Here's the drawing with two shaded views (mm, measured from the low corner). I have some questions. Coordinates: 2 decimals unless noted, no trailing zeros. Loops run counter-clockwise (first coordinate to the right, second up) from the corner with the lowest first, then second, coordinate; pieces in that order, holes last.
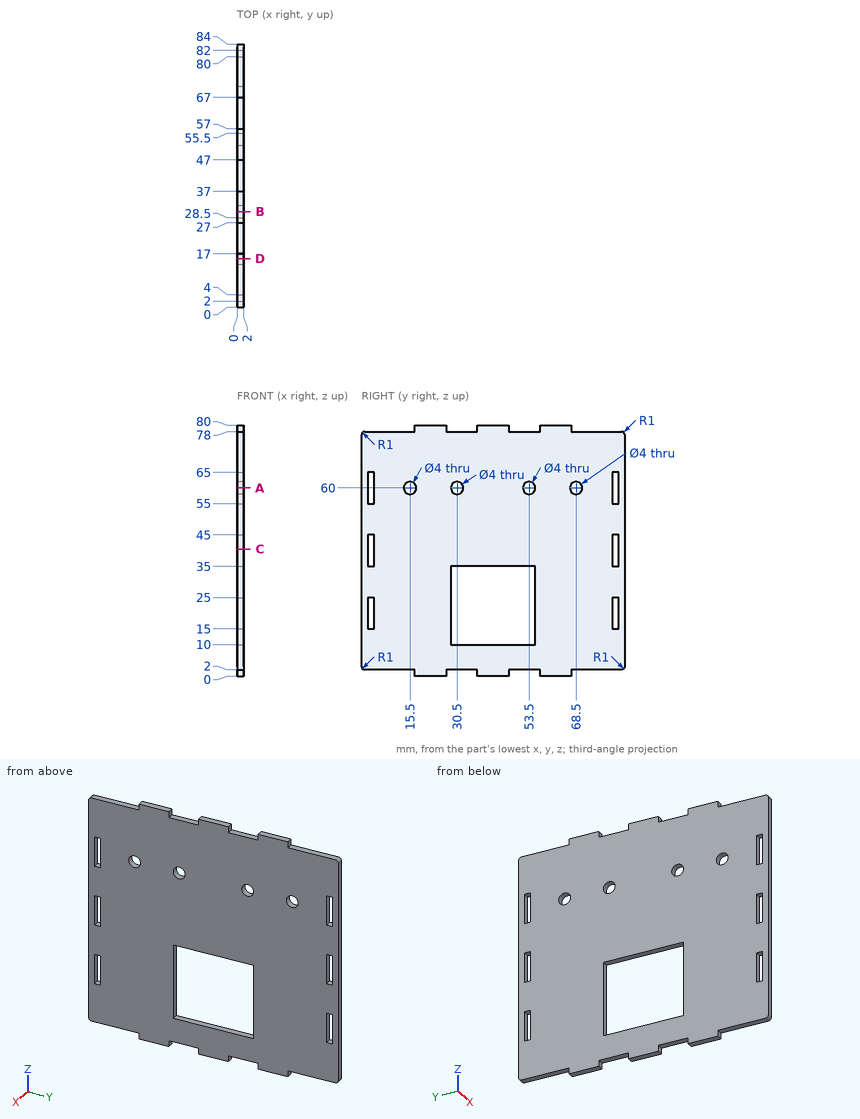
Q1. Suppose I cut it at C-C on z = 40.5. Write out the boundary of the cut face in (x, y), and give its area (3 significant figures).
Q2. Suppose I cut it at A-A on z = 60. Write out the boundary of the cut face in (x, y), and give its area (3 significant figures).
Q3. Will these pins go through, and if not, where does the flat tip stop? P1, Ø1, axis at x = 1, y = 78, coming from the +Z side; P2, Ø1, axis at x = 1.5, z = 1, coming from the -Y side; P3, Ø1, axis at x = 1, z = 79.5, coming from the +Y side.
Q4. Please list where these lines run through material, in increasing order: probe 1 along Z at (x, y) = (0.8, 53.5); probe 2 along Y at (x, z) = (0.5, 64); probe 3 along Y at (x, z) = (0.5, 27).
Q5. Suppose I cut it at B-B on y = 30.5. Write out the boundary of the cut face in (x, z).
Q6. Suppose I cut it at D-D on y = 15.5. Write out the boundary of the cut face in (x, z).
Check values:
1. outline: (0, 0) - (2, 0) - (2, 2) - (0, 2) - close; (0, 4) - (2, 4) - (2, 80) - (0, 80) - close; (0, 82) - (2, 82) - (2, 84) - (0, 84) - close
1. area: 160 mm2
2. outline: (0, 0) - (2, 0) - (2, 2) - (0, 2) - close; (0, 4) - (2, 4) - (2, 13.5) - (0, 13.5) - close; (0, 17.5) - (2, 17.5) - (2, 28.5) - (0, 28.5) - close; (0, 32.5) - (2, 32.5) - (2, 51.5) - (0, 51.5) - close; (0, 55.5) - (2, 55.5) - (2, 66.5) - (0, 66.5) - close; (0, 70.5) - (2, 70.5) - (2, 80) - (0, 80) - close; (0, 82) - (2, 82) - (2, 84) - (0, 84) - close
2. area: 128 mm2
3. P1: stops at z = 78
3. P2: stops at y = 17
3. P3: stops at y = 67
4. probe 1: z = 2 to 10, 35 to 58, 62 to 78
4. probe 2: y = 0 to 2, 4 to 80, 82 to 84
4. probe 3: y = 0 to 28.5, 55.5 to 84
5. outline: (0, 2) - (2, 2) - (2, 10) - (0, 10) - close; (0, 35) - (2, 35) - (2, 58) - (0, 58) - close; (0, 62) - (2, 62) - (2, 78) - (0, 78) - close
6. outline: (0, 2) - (2, 2) - (2, 58) - (0, 58) - close; (0, 62) - (2, 62) - (2, 78) - (0, 78) - close
